Design review of the part built by this model. Coordinates are the model's own, in mm. Face numbers are marked on the shaded views. Coordinates: 2 decimals unless noted, no trailing zeros. Loops run counter-clockwise (first coordinate to the right, second up) from the corner with the lowest first, then second, coordinate; pieces in that order, holes last. Notation, with made-up numbers: (51, 8.25) - (84, 8.25) arc R21 ccw to (84, 16.25) - close; hole circle Ø7 at (-13.5, 65). An arc over 180 degrees is marked (long way). Use one line per item in the form item = value. Start each with the question number.
(1) Clearance check with flat-ended pins moving along their axes: pin 1 Ø6 at (y, z) = (13, 91) entering from +X; pin 2 Ø4 at (x, y) = (9.5, 2) entering from -Z; pin 3 Ø5 at (x, y) = (26, -4.5) entering from +Z. State where each tip first meets the part, or that it passes through.
(2) For L1, parallel to Z at x = 65.8, y = 0; L2, parallel to X at y = 0, z = 75; L3, parallel to Y at x = 31.5, z = 40.5, list the stretches that pass through material, from the lowest coordinate up.
(3) Add section C-C (z = 5). State the section outline as (x, y) points, plus the area to 3 significant figures.
(4) Add section D-D (y = 14.5). State the section outline as (x, z) points, plus the area to 3 significant figures.
(5) Add section A-A (x = 32.5). State the section outline as (y, z) points.
(6) The part is to be moulded in two halves that separate along X. For the marked faces 1 and 2, say which applies: pulls with the +X half, pulls with the -X half, needs draft (parallel to the pull), parting line crosses it, or undercut.
(7) Add section B-B (y = 0). State the section outline as (x, z) points.
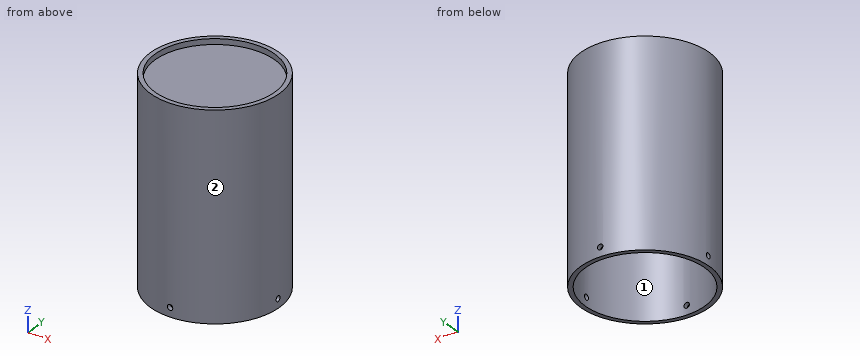
Autodesk Inventor part; units mm, degrees
ref_plane "YZ Plane" through (0, 0, 0) normal (1, 0, 0) x (0, 1, 0)
ref_plane "XZ Plane" through (0, 0, 0) normal (0, 1, 0) x (-1, 0, 0)
ref_plane "XY Plane" through (0, 0, 0) normal (0, 0, 1) x (1, 0, 0)
sketch "Sketch1" plane through (0, 0, 0) normal (0, 1, 0) x (-1, 0, 0)
  line L0 (-67.5, -60) -> (-67.5, 0)
  line L1 (2.5, -60) -> (2.5, 0)
  line L2 (-67.5, 0) -> (2.5, 0)
  line L3 (-32.5, 0) -> (-32.5, 110)
  line L4 (2.5, -60) -> (-67.5, -60)
  line L5 (-67.5, 0) -> (-67.5, 110)
  line L6 (-65, 0) -> (-65, -30)
  line L7 (0, 0) -> (0, -30)
  line L8 (-65, 0) -> (-65, 110)
  line L9 (-65, 110) -> (-67.5, 110)
  line L10 (-65, 0) -> (-67.5, 0)
  line L11 (-65, 107) -> (-32.5, 107)
  line L12 (-32.5, 107) -> (-32.5, 102)
  line L13 (-32.5, 102) -> (-65, 102)
  line L14 (-65, 102) -> (-65, 107)
  dimension "d1" = 170
  dimension "d2" = 5
  dimension "d3" = 3
revolve "Revolution1" add sketch "Sketch1" angle 360 about axis through (32.5, 0, 0) along (0, 0, 1) contours L5 L9 L8 L2 | L8 L11 L3 L13
sketch "Sketch2" plane through (0, 0, 0) normal (0, 1, 0) x (-1, 0, 0)
  line L0 (2.5, 0) -> (-67.5, 0)
  line L1 (2.5, 110) -> (-67.5, 110)
  line L2 (-32.5, 0) -> (-32.5, 5)
  circle A0 centre (-32.5, 5) radius 1.5
  point P0 (0, 0)
  dimension "d5" = 5
  dimension "d6" = 3
extrude "Extrusion1" cut sketch "Sketch2" along normal through all both and the other way through all
sketch "Sketch3" plane through (0, 0, 0) normal (1, 0, 0) x (0, 1, 0)
  line L0 (35, 0) -> (-35, 0)
  line L1 (35, 110) -> (-35, 110)
  line L2 (0, 0) -> (0, 5)
  circle A0 centre (0, 5) radius 1.5
  point P0 (34.9678, 5)
  point P1 (-34.9678, 5)
  dimension "d9" = 5
  dimension "d10" = 3
extrude "Extrusion2" cut sketch "Sketch3" along normal through all both and the other way through all
properties part number "GrundkörperOben"
Computed values:
q1.pin_1 = 66.04
q1.pin_2 = 102
q1.pin_3 = 107
q2.L1 = 0 to 3.5, 6.5 to 110
q2.L2 = -2.5 to 0, 65 to 67.5
q2.L3 = -34.99 to -32.48, 32.48 to 34.99
q3.outline = (-2.47, -1.5) arc R35 ccw to (31, -34.97) - (31, -32.47) arc R32.5 cw to (0.03, -1.5) - close; (-2.47, 1.5) - (0.03, 1.5) arc R32.5 cw to (31, 32.47) - (31, 34.97) arc R35 ccw to start; (34, -34.97) arc R35 ccw to (67.47, -1.5) - (64.97, -1.5) arc R32.5 cw to (34, -32.47) - close; (34, 32.47) arc R32.5 cw to (64.97, 1.5) - (67.47, 1.5) arc R35 ccw to (34, 34.97) - close
q3.area = 500 mm^2
q4.outline = (0.64, 0) - (3.41, 0) - (3.41, 102) - (61.59, 102) - (61.59, 0) - (64.36, 0) - (64.36, 110) - (61.59, 110) - (61.59, 107) - (3.41, 107) - (3.41, 110) - (0.64, 110) - close
q4.area = 900 mm^2
q5.outline = (-35, 0) - (-32.5, 0) - (-32.5, 3.5) - (-35, 3.5) - close; (-35, 6.5) - (-32.5, 6.5) - (-32.5, 102) - (32.5, 102) - (32.5, 6.5) - (35, 6.5) - (35, 110) - (32.5, 110) - (32.5, 107) - (-32.5, 107) - (-32.5, 110) - (-35, 110) - close; (32.5, 0) - (35, 0) - (35, 3.5) - (32.5, 3.5) - close
q6.face_1 = undercut
q6.face_2 = parting line crosses it
q7.outline = (-2.5, 0) - (0, 0) - (0, 3.5) - (-2.5, 3.5) - close; (-2.5, 6.5) - (0, 6.5) - (0, 102) - (65, 102) - (65, 6.5) - (67.5, 6.5) - (67.5, 110) - (65, 110) - (65, 107) - (0, 107) - (0, 110) - (-2.5, 110) - close; (65, 0) - (67.5, 0) - (67.5, 3.5) - (65, 3.5) - close
